from build123d import *

# Parameters (mm, degrees)
F0_W     = 545
F0_H     = 350
F0_W_2   = 475
F0_H_2   = 340
F1_DEPTH = 149
F3_W     = 545
F3_H     = 350
F4_DEPTH = 5
F5_D     = 4
F5_DEPTH = 15
F5_TIP   = 1.2017212381


with BuildPart() as f1:
    # F0 (on Top) → F1 (new body, symmetric)
    with BuildSketch(Plane.XY):
        Rectangle(F0_W, F0_H)
        Rectangle(F0_W_2, F0_H_2, mode=Mode.SUBTRACT)
    extrude(amount=F1_DEPTH, both=True)

    # F3 (on face) → F4 (join)
    with BuildSketch(Plane(origin=(0, 0, -149), x_dir=(1, 0, 0), z_dir=(0, 0, -1))):
        Rectangle(F3_W, F3_H)
    extrude(amount=F4_DEPTH)

    # F5
    with Locations(Plane.YZ.offset(272.5)):
        with Locations((-12.5, 89), (12.5, 89), (-12.5, -21), (12.5, -21)):
            Hole(F5_D / 2, depth=F5_DEPTH)
            with Locations((0, 0, -(F5_DEPTH + F5_TIP / 2))):  # 118° drill point
                Cone(0, F5_D / 2, F5_TIP, mode=Mode.SUBTRACT)


solid = f1.part
Source: CAD feature listing. Evaluate the final solid. Frame: model axes, mm. A direction names the side the tool comes from. Coordinates: 2 decimals unless noted, no trailing zeros. Loops run counter-clockwise (first coordinate to the right, second up) from the corner with the lowest first, then second, coordinate; pieces in that order, holes last. Notation, with made-up numbers: (55.5, 21) - (62.5, 21) arc R32 ccw to (62.5, 58) - close; hole circle Ø11 at (-5.5, 10.25). An arc over 180 degrees is marked (long way). Return JSON: item names as keys, results as strings.
Q1. Section A-A, the plane z = -5.5. Return loops of the section in (x, y).
Results:
{"outline": "(-272.5, -175) - (272.5, -175) - (272.5, 175) - (-272.5, 175) - close; hole (-237.5, -170) - (237.5, -170) - (237.5, 170) - (-237.5, 170) - close"}
Q2. Access query for faces 4 (the flat face through (-272.5, 2, 0)), 5 (the flat face through (-3, -170, 2)). Directions: +Z, -Z, +X, -X, +Y, -Y. A direction counts if a zero-diameter tool reaches every point of the face in a straight line with its end or side. Return the directions, or none.
Results:
{"face 4": "+Z, -Z, -X, +Y, -Y", "face 5": "+Z"}
Q3. Material intervals for line 1 along Y through (x, z) = (268, -21); line 2 along X through (y, z) = (135, 5); line 3 along Y through (x, z) = (-134, 102.5), sorted ascending.
Results:
{"line 1": "-175 to -14.5, -10.5 to 10.5, 14.5 to 175", "line 2": "-272.5 to -237.5, 237.5 to 272.5", "line 3": "-175 to -170, 170 to 175"}
Q4. Section C-C, the plane x = -90. Return loops of the section in (y, z), plus the area to 3 significant figures.
Results:
{"outline": "(-175, -154) - (175, -154) - (175, 149) - (170, 149) - (170, -149) - (-170, -149) - (-170, 149) - (-175, 149) - close", "area": "4,730 mm2"}
Q5. Mould query, pull axis Y, two halves, no side actions, for faces 1 (the flat face through (-4, -175, 0)), 2 (the flat face through (-4, -2, -154)), 3 (the flat face through (237.5, -2, 2)). Classes: released by +Y, released by -Y, zero draft, split by the parting line, or undercut.
Results:
{"face 1": "released by -Y", "face 2": "zero draft", "face 3": "undercut"}
Q6. Section B-B, the plane y = 148.5. Return loops of the section in (x, z), plus the area to 3 significant figures.
Results:
{"outline": "(-272.5, -154) - (272.5, -154) - (272.5, 149) - (237.5, 149) - (237.5, -149) - (-237.5, -149) - (-237.5, 149) - (-272.5, 149) - close", "area": "23,600 mm2"}
Q7. Contact query for a flat-ended pin moving along its axis: P1, Ø5, axis at x = -84.5, y = 116, coming from the +Z side. Output: stop coordinate, or through.
Results:
{"P1": "z = -149"}
